Can you work these out from the model? Positions are in its coordinate system, mm. Face numbers are marked on the shaded views. Coordinates: 2 decimals unless noted, no trailing zeros. Order: outer loops, then holes, each group sorted by start corner. A loop starts at its lowest first (then second) coordinate and runs counter-clockwise, first axis right, second up. Notation, with made-up numbers: (9.25, -18) -> (22.25, -18) arc R17 ccw to (22.25, -11) -> close; hole circle Ø4 at (79, 80). An arc over 180 degrees is marked (long way). Return JSON: item names as keys, results as strings. Group by question number.
1) For pin 1 (8 mm diameter, centred on x = -13.5, z = 10.5, fed in from -Y); pin 2 (1.5 mm diameter, centred on x = 1, y = 4, fed in from +Z); pin 3 (10 mm diameter, centred on x = 0.5, z = 5.5, fed in from +Y), each with a flat end and sliding along its axis, tell me the tip position at first contact or that it passes through.
2) Thinking about a two-plate mould opening in Y: for the marked faces 1, 2 and 3, which applies, +Y half, -Y half, draft (parallel to the pull), parting line (faces both ways), or undercut?
3) If we section it at B-B, the plane z = 13.25: Please give me the cut outline in (x, y).
4) If we section it at A-A, the plane z = 7.75: Please give me the cut outline in (x, y), then the cut area to 3 significant figures.
5) If I drill on probe 1 along Y at (x, z) = (-28.5, 10.5); probe 2 along X at (y, z) = (23, 11); probe 3 along Z at (x, y) = (-25.5, 0), over which ranges is the centre line in solid material (lowest first)? Write a range as from..to.
from build123d import *

# Parameters (mm, degrees)
BOSS_EXTRUDE1_OUTLINE_R = 10.616834944
BOSS_EXTRUDE1_DEPTH     = 3
SKETCH3_R               = 40
SKETCH3_R_2             = 37
BOSS_EXTRUDE2_DEPTH     = 15
SKETCH4_R               = 11.616834944
SKETCH4_R_2             = 10.616834944
BOSS_EXTRUDE3_DEPTH     = 2
FILLET2_R               = 2
FILLET3_R               = 6
SKETCH6_R               = 2.38125
CUT_EXTRUDE1_DEPTH      = 3.175
SKETCH8_R               = 4.38125
BOSS_EXTRUDE5_DEPTH     = 1


# Read off the part's stored shape, not the designer's step: Boss-Extrude1
with BuildPart() as part:
    # Boss-Extrude1 outline → Boss-Extrude1 (new body)
    with BuildSketch(Plane.XY):
        with BuildLine():
            Line((-61.158014619, -0.130841154), (-60.258391765, -0.130841154))
            ThreePointArc((-60.258391765, -0.130841154), (-28.255886619, -16.129333036), (3.743709339, -0.125023097))
            ThreePointArc((3.743709339, -0.125023097), (6.087180251, 0.966663669), (7.041985381, 3.369158846))
            Line((7.041985381, 3.369158846), (7.041985381, 5.061001168))
            ThreePointArc((7.041985381, 5.061001168), (-31.332414811, 63.752458818), (-60.262892503, -0.124839588))
            ThreePointArc((-60.262892503, -0.124839588), (-62.604293531, 0.967812618), (-63.558014619, 3.369158846))
            Line((-63.558014619, 3.369158846), (-63.558014619, 2.269158846))
            ThreePointArc((-63.558014619, 2.269158846), (-62.855070894, 0.572102571), (-61.158014619, -0.130841154))
        make_face()
        with Locations((-28.259522786, 23.870666799)):
            Circle(BOSS_EXTRUDE1_OUTLINE_R, mode=Mode.SUBTRACT)
    extrude(amount=BOSS_EXTRUDE1_DEPTH)

    # Sketch3 → Boss-Extrude2 (add)
    with BuildSketch(Plane.XY.offset(3)):
        with Locations(Location((-28.259522786, 23.870666799, 0), (0, 0, 216.861852286))):
            Circle(SKETCH3_R)
        with Locations((-28.259522786, 23.870666799)):
            Circle(SKETCH3_R_2, mode=Mode.SUBTRACT)
    extrude(amount=BOSS_EXTRUDE2_DEPTH)

    # Sketch4 → Boss-Extrude3 (add)
    with BuildSketch(Plane.XY.offset(3)):
        with Locations((-28.259522786, 23.870666799)):
            Circle(SKETCH4_R)
        with Locations((-28.259522786, 23.870666799)):
            Circle(SKETCH4_R_2, mode=Mode.SUBTRACT)
    extrude(amount=BOSS_EXTRUDE3_DEPTH)

    # Fillet2
    fillet2_edges = [part.edges().sort_by_distance(p)[0] for p in [
        (-39.87635773, 23.870666799, 3),
    ]]
    fillet(fillet2_edges, radius=FILLET2_R - 0.0001)  # a hair under: the kernel refuses the full size

    # Fillet3
    fillet3_edges = [part.edges().sort_by_distance(p)[0] for p in [
        (-65.259522786, 23.870666799, 3),
    ]]
    fillet(fillet3_edges, radius=FILLET3_R)

    # Sketch6 → Cut-Extrude1 (cut)
    with BuildSketch(Plane(origin=(0, 0, 0), x_dir=(-1, 0, 0), z_dir=(0, 0, -1))):
        with Locations((58.558014619, 4.869158846)):
            Circle(SKETCH6_R)
        with Locations((58.558014619, 33.869158846)):
            Circle(SKETCH6_R)
        with Locations((-2.041985381, 33.869158846)):
            Circle(SKETCH6_R)
        with Locations((-2.041985381, 4.869158846)):
            Circle(SKETCH6_R)
    extrude(amount=-CUT_EXTRUDE1_DEPTH, mode=Mode.SUBTRACT)

    # Sketch8 → Boss-Extrude5 (add)
    with BuildSketch(Plane(origin=(0, 0, 3), x_dir=(-1, 0, 0), z_dir=(0, 0, -1))):
        with Locations((58.558014619, 4.869158846)):
            Circle(SKETCH8_R)
        with Locations((58.558014619, 33.869158846)):
            Circle(SKETCH8_R)
        with Locations((-2.041985381, 33.869158846)):
            Circle(SKETCH8_R)
        with Locations((-2.041985381, 4.869158846)):
            Circle(SKETCH8_R)
    extrude(amount=-BOSS_EXTRUDE5_DEPTH)


solid = part.part
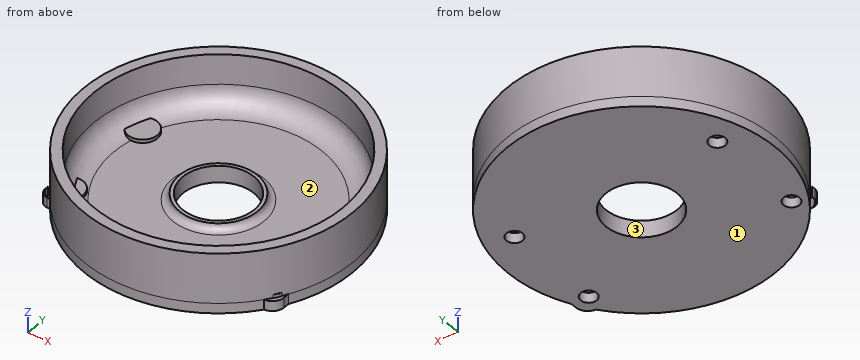
Result sheet:
{
 "1": {"pin 1": "stops at y = -14.66", "pin 2": "stops at z = 5.87", "pin 3": "stops at y = 56.05"},
 "2": {"face 1": "draft", "face 2": "undercut", "face 3": "undercut"},
 "3": {"outline": "circle Ø80 at (-28.26, 23.87); hole circle Ø74 at (-28.26, 23.87)"},
 "4": {"outline": "circle Ø80 at (-28.26, 23.87); hole circle Ø73.74 at (-28.26, 23.87)", "area": "756 mm2"},
 "5": {"probe 1": "y = -16.13..-13.13, 60.87..63.87", "probe 2": "x = -68.25..-65.25, 8.73..11.73", "probe 3": "z = 0..3"}
}
